Answer from the drawing. Dimensions are ordinates in mm from the lowest x, y and z of the part. A direction names the side the tool comes from. Round coordinates to 2 decimals unless told otherwise and drop trailing zeros. Write each loop counter-clockwise with the first axis right and the second up, starting at its lowest first coordinate (ties: lowest second). Pieces come first, ordered by that corner, then holes. Notation, with made-up numbers: (-16, 30) - (33, 30) arc R9 cw to (33, 46) - close; hole circle Ø10 at (30, 16). An arc over 180 degrees is marked (long way). One line per item, written item: value. Start each with the question number.
(1) The mould has two halves that part along Y. Classify the marked faces 1 and 2: +Y half, -Y half, draft (parallel to the pull), parting line (faces both ways), or undercut.
(2) For the marked faces 3 and 4, determine the directions among +Z, -Z, +X, -X, +Y, -Y from which every point of the face is accessible in a straight line to the end or side of a thin tool.
(3) A cutting plane is placed at B-B, the plane z = 3.75. Determine the outline of the cut face in (x, y).
(4) Flat-ended cylindrical pins translate along their axes: pin 1 Ø2 at (x, z) = (10.5, 3.5) entering from -Y; pin 2 Ø1.6 at (x, z) = (11, 3.5) entering from +Y; pin 3 Ø1.4 at (x, y) = (11.1, 1.8) entering from -Z; pin 4 Ø1.6 at (y, z) = (6, 3.5) entering from -X. Find the tip coordinate at first contact, or state that the pin passes through.
(5) A cutting plane is placed at D-D, the plane x = 2.1. Determine the outline of the cut face in (y, z).
(6) A cutting plane is placed at A-A, the plane x = 7.5. Determine the outline of the cut face in (y, z), plus the area to 3 significant figures.
(7) Find the intervals of material crossed by L1, parallel to Y at x = 2.1, z = 2.1; L2, parallel to Y at x = 11.1, z = 2; L3, parallel to Y at x = 6.5, z = 1.2, in increasing order.
(8) A cutting plane is placed at C-C, the plane z = 1.45. Determine the outline of the cut face in (x, y).
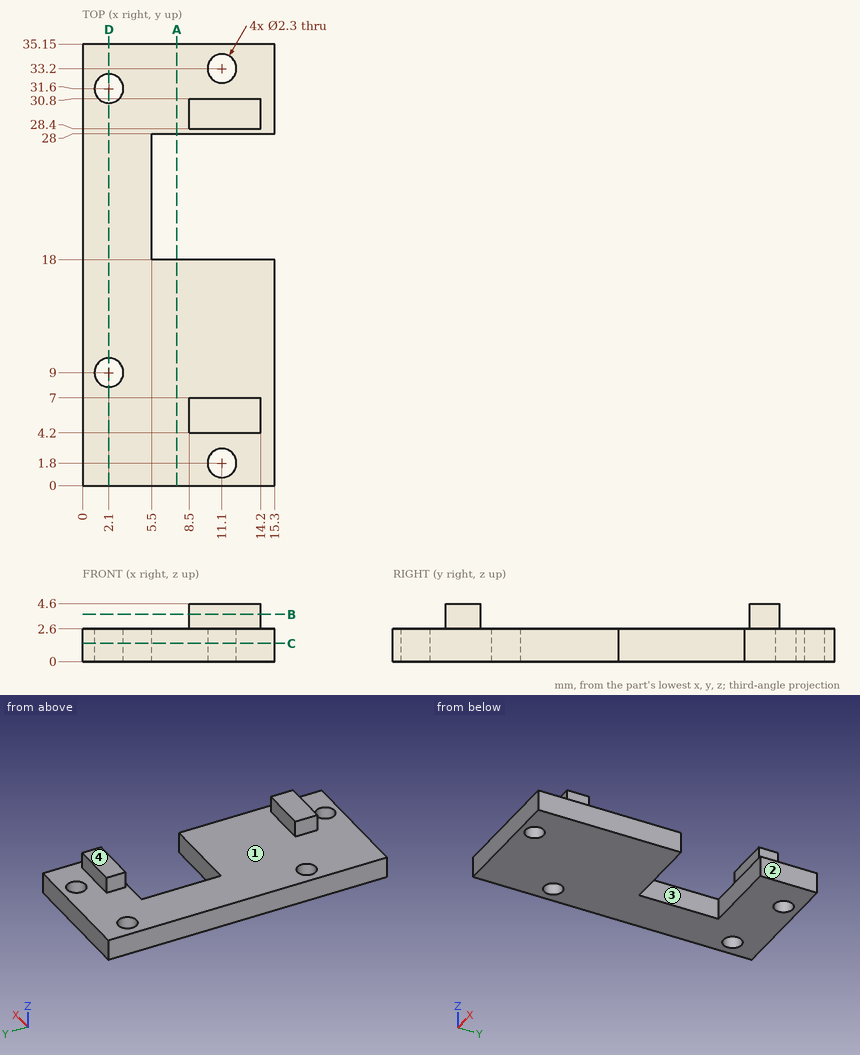
Here are the results:
1. face 1: undercut
1. face 2: draft
2. face 3: +Z, -Z, +X
2. face 4: +Z, +X, -X, +Y, -Y
3. outline: (8.5, 4.2) - (14.2, 4.2) - (14.2, 7) - (8.5, 7) - close; (8.5, 28.4) - (14.2, 28.4) - (14.2, 30.8) - (8.5, 30.8) - close
4. pin 1: y = 0
4. pin 2: y = 30.8
4. pin 3: through
4. pin 4: x = 8.5
5. outline: (0, 0) - (7.85, 0) - (7.85, 2.6) - (0, 2.6) - close; (10.15, 0) - (30.45, 0) - (30.45, 2.6) - (10.15, 2.6) - close; (32.75, 0) - (35.15, 0) - (35.15, 2.6) - (32.75, 2.6) - close
6. outline: (0, 0) - (18, 0) - (18, 2.6) - (0, 2.6) - close; (28, 0) - (35.15, 0) - (35.15, 2.6) - (28, 2.6) - close
6. area: 65.4 mm²
7. L1: 0 to 7.85, 10.15 to 30.45, 32.75 to 35.15
7. L2: 0 to 0.65, 2.95 to 18, 28 to 32.05, 34.35 to 35.15
7. L3: 0 to 18, 28 to 35.15
8. outline: (0, 0) - (15.3, 0) - (15.3, 18) - (5.5, 18) - (5.5, 28) - (15.3, 28) - (15.3, 35.15) - (0, 35.15) - close; hole circle Ø2.3 at (2.1, 9); hole circle Ø2.3 at (2.1, 31.6); hole circle Ø2.3 at (11.1, 1.8); hole circle Ø2.3 at (11.1, 33.2)
